The listing builds one solid part. Answer for the finished solid, in the listing's coordinates (mm). Face numbers are marked on the shaded views. A direction names the side the tool comes from. Coordinates: 2 decimals unless noted, no trailing zeros. Write each loop counter-clockwise with the first axis right and the second up, starting at its lowest first coordinate (ties: lowest second). Pieces come first, ordered by that corner, then holes. Notation, with made-up numbers: M 0.5,70 L 8.5,70 A18 ccw 8.5,83 Z; hole C 63.5,-3.75 d5. An arc over 180 degrees is marked long. Answer as CSV lines item,"result".
```python
from build123d import *

# Parameters (mm, degrees)
F0_W     = 25.4
F0_H     = 19.05
F1_DEPTH = 25.4
F2_DEPTH = 63.5
F3_DEPTH = 7.9375
F5_R     = 6.35


with BuildPart() as f1:
    # F0 (on Front) → F1 (new body, symmetric)
    with BuildSketch(Plane.XZ):
        with Locations((73.025, 52.4002)):
            Rectangle(F0_W, F0_H)
        with BuildLine():
            Line((22.225, 27.0002), (22.225, 9.525))
            Line((22.225, 9.525), (41.275, 9.525))
            Line((41.275, 9.525), (41.275, 27.0002))
            ThreePointArc((41.275, 27.0002), (45.9246798487, 38.2255201513), (57.15, 42.8752))
            Line((57.15, 42.8752), (60.325, 42.8752))
            Line((60.325, 42.8752), (60.325, 61.9252))
            Line((60.325, 61.9252), (57.15, 61.9252))
            add(Edge.make_bspline(
                [(57.15, 61.9252), (56.7952901296, 61.9213576462), (56.4397740543, 61.9159247713), (56.0834888873, 61.9089120795)],
                knots=[0, 0, 0, 0, 0.9203452137, 0.9203452137, 0.9203452137, 0.9203452137], degree=3))
            ThreePointArc((56.0834888873, 61.9089120795), (32.0800625688, 51.3159122494), (22.225, 27.0002))
        make_face()
    extrude(amount=F1_DEPTH, both=True)

    # F0 (on Front) → F2 (join, symmetric)
    with BuildSketch(Plane.XZ):
        Polygon((22.225, 9.525), (-41.275, 9.525), (-41.275, -9.525), (41.275, -9.525), (41.275, 9.525), align=None)
    extrude(amount=F2_DEPTH, both=True)

    # F0 (on Front) → F3 (join, symmetric)
    with BuildSketch(Plane.XZ):
        with BuildLine():
            add(Edge.make_bspline(
                [(56.0834888873, 61.9089120795), (13.2740013728, 61.0663012405), (-40.6390568029, 37.4154732137), (-41.275, 9.525)],
                knots=[0.9203452137, 0.9203452137, 0.9203452137, 0.9203452137, 111.5045361635, 111.5045361635, 111.5045361635, 111.5045361635], degree=3))
            Line((-41.275, 9.525), (22.225, 9.525))
            Line((22.225, 9.525), (22.225, 27.0002))
            ThreePointArc((22.225, 27.0002), (32.0800625688, 51.3159122494), (56.0834888873, 61.9089120795))
        make_face()
    extrude(amount=F3_DEPTH, both=True)

    # F0 (on Front) → F4 (revolve)
    with BuildSketch(Plane.XZ):
        Polygon((85.725, 66.675), (85.725, 61.9252), (85.725, 42.8752), (85.725, 34.925), (111.125, 34.925), (111.125, 66.675), align=None)
    revolve(axis=Axis((85.725, 0, 50.8), (0, 0, 1)))

    # F5
    f5_edges = [f1.edges().sort_by_distance(p)[0] for p in [
        (41.275, -63.5, 0),
        (-41.275, -63.5, 0),
        (41.275, 63.5, 0),
        (-41.275, 63.5, 0),
    ]]
    fillet(f5_edges, radius=F5_R)


solid = f1.part
```
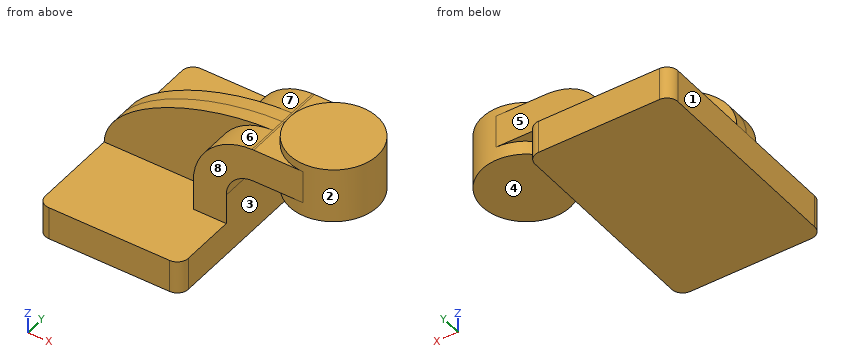
Q1. For the marked faces 5, 6, 7 and 8, determine the directions among +Z, -Z, +X, -X, +Y, -Y from which every point of the face is accessible in a straight line to the end or side of a thin tool.
Output:
face 5,"+Z, +X, -X, +Y"
face 6,"+Z, -X, -Y"
face 7,"+Z, -X, +Y"
face 8,"+Z, +X, -X, -Y"
Q2. Straight lines are drawn through the part: line 1 (Z direction, x = 26, y = -53.5) (3 decimals); line 2 (X direction, y = 9, z = 2) (3 decimals); line 3 (Y direction, x = -9.5, z = 23). For each, find the intervals that lie inside material, in ascending order.
Output:
line 1,"-9.525 to 9.525"
line 2,"-41.275 to 41.275"
line 3,"-7.94 to 7.94"
Q3. The mould has two halves that part along X. Classify the marked faces 1, 2, 3 and 4: pulls with the +X half, pulls with the -X half, needs draft (parallel to the pull), parting line crosses it, or undercut.
Output:
face 1,"pulls with the -X half"
face 2,"undercut"
face 3,"pulls with the +X half"
face 4,"needs draft"
Q4. Flat-ended cylindrical pins translate along their axes: pin 1 Ø5 at (y, z) = (-15, 20.5) entering from -X (3 decimals); pin 2 Ø16.5 at (x, y) = (7.5, -25) entering from +Z (3 decimals); pin 3 Ø12 at (y, z) = (-25.5, 34) entering from +X; pin 4 Ø10 at (x, z) = (46.5, 25) entering from +Y. Find the tip coordinate at first contact, or state that the pin passes through.
Output:
pin 1,"x = 22.225"
pin 2,"z = 9.525"
pin 3,"x = 101.91"
pin 4,"through"
Q5. Find section B-B (x = 92). Give the vertices of the cut face in (y, z) (3 decimals).
Output:
outline,"M -24.613,34.925 L 24.613,34.925 L 24.613,66.675 L -24.613,66.675 Z"
Q6. Find section A-A (y = -45). Give the vertices of the cut face in (x, z) (3 decimals).
Output:
outline,"M -41.275,-9.525 L 41.275,-9.525 L 41.275,9.525 L -41.275,9.525 Z"
